Model file for the job. Use its own axes, mm. Face numbers are marked on the shaded views. A direction names the side the tool comes from. Coordinates: 2 decimals unless noted, no trailing zeros. Order: outer loops, then holes, each group sorted by start corner. A loop starts at its lowest first (then second) coordinate and runs counter-clockwise, first axis right, second up. Notation, with made-up numbers: M 23.25,-39.5 L 72.25,-39.5 A31 cw 72.25,-6.5 Z; hole C 12,0 d11. An arc over 180 degrees is marked long. Return JSON: item names as keys, results as strings.
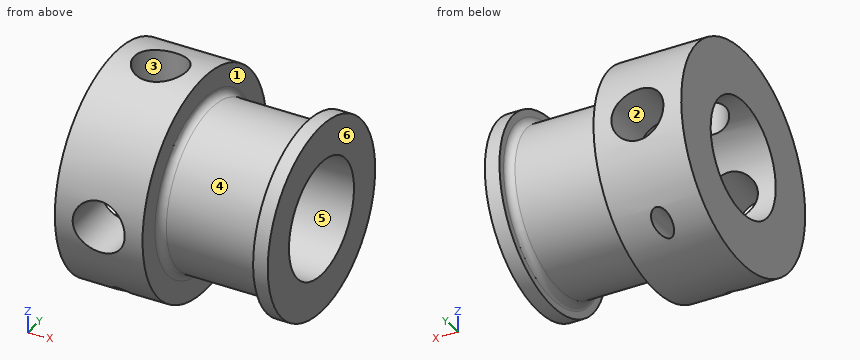
```python
from build123d import *

# Parameters (mm, degrees)
SKETCH1_R            = 4.7625
SKETCH1_R_2          = 2.499995
BASE_DEPTH           = 8.89
CRIMPHOLE_DEPTH      = 12.153246725
CRIMPHOLE_DEPTH_BACK = 12.153246725
SKETCH7_R            = 0.396875
SKETCH3_W            = 1.1303
SKETCH3_H            = 4.7635
CUTTERRAD_R          = 0.3175
CIRPATTERN1_COUNT    = 4


with BuildPart() as part:
    # Sketch1 → Base (new body)
    with BuildSketch(Plane(origin=(0, 0, 0), x_dir=(0, 0, -1), z_dir=(1, 0, 0))):
        Circle(SKETCH1_R)
        Circle(SKETCH1_R_2, mode=Mode.SUBTRACT)
    extrude(amount=BASE_DEPTH)

    # Sketch2 → Spool (revolve, cut)
    with BuildSketch(Plane.XY, mode=Mode.PRIVATE) as spool_sk:
        Polygon((3.81, 4.7625), (8.89, 4.7625), (8.89, 4.1275), (8.255, 4.1275), (8.255, 3.4925), (3.81, 3.4925), align=None)
    revolve(spool_sk.sketch.rotate(Axis((8.89, 0, 0), (-1, 0, 0)), 90), axis=Axis((8.89, 0, 0), (-1, 0, 0)), mode=Mode.SUBTRACT)

    # Sketch7 → CrimpHole (cut, two sides: drawn at the far end of the back side and taken through both)
    with BuildSketch(Plane(origin=(0, 0, 0), x_dir=(1, 0, 0), z_dir=(0, 1, 0)).offset(-CRIMPHOLE_DEPTH_BACK)):
        with Locations(Location((1.905, 3.81, 0), (0, 0, 270))):
            Circle(SKETCH7_R)
    extrude(amount=CRIMPHOLE_DEPTH + CRIMPHOLE_DEPTH_BACK, mode=Mode.SUBTRACT)

    # Sketch3 → ShaftSetScrew (revolve, cut)
    with BuildSketch(Plane.YZ.offset(1.905)):
        with Locations((0.56515, 2.38175)):
            Rectangle(SKETCH3_W, SKETCH3_H)
    shaftsetscrew = revolve(axis=Axis((1.905, 0, -6.35), (0, 0, 1)), mode=Mode.SUBTRACT)

    # CutterRad
    cutterrad_edges = [part.edges().sort_by_distance(p)[0] for p in [
        (3.81, 0, 3.4925),
        (8.255, 0, 3.4925),
    ]]
    fillet(cutterrad_edges, radius=CUTTERRAD_R)

    # CirPattern1: ShaftSetScrew ×4 about axis, 1 skipped
    cirpattern1_axis = Axis((8.89, 0, 0), (-1, 0, 0))
    add([shaftsetscrew.rotate(cirpattern1_axis, i * 360 / CIRPATTERN1_COUNT) for i in range(1, CIRPATTERN1_COUNT) if i not in (2,)], mode=Mode.SUBTRACT)


solid = part.part
```
Item 1: Saw through at A-A (z = 0). Count the separate pieces of the cut face and the enclosed holes in it, and give its area (3 significant figures).
Check result:
{"separate pieces": "4", "enclosed holes": "0", "area": "18.0 mm2"}
Item 2: 3-axis set-ups, long thin cutter, end or side, ignore diameter. For the marked faces 1 and 2: which of +Z, -Z, +X, -X, +Y, -Y reach the whole face in a straight line?
Check result:
{"face 1": "none", "face 2": "+Y, -Y"}
Item 3: Wall check: line 1 (Y direction, x = 3.75, z = 0); line 2 (X direction, y = -2.75, z = 0); line 3 (Y direction, x = 4.25, z = 1). Give the ranges that are in metal, low to high.
Check result:
{"line 1": "y = -4.76 to -2.5, 2.5 to 4.76", "line 2": "x = 0 to 0.77, 3.04 to 8.89", "line 3": "y = -3.35 to -2.29, 2.29 to 3.35"}
Item 4: Pull direction Y, two halves, no side cores. Call the marked faces 3, 4, 5 and 6: +Y half, -Y half, draft (parallel to the pull), parting line (faces both ways), or undercut.
Check result:
{"face 3": "undercut", "face 4": "parting line", "face 5": "undercut", "face 6": "draft"}
Item 5: Saw through at B-B (x = 4.75). Write the cut outline in (y, z) (1 decimal).
Check result:
{"outline": "C 0,0 d7; hole C 0,0 d5"}
Item 6: Drop flat-ended pins along their axis: pin 1 Ø1 at (x, z) = (1.5, -1) entering from +Y; pin 2 Ø1.5 at (x, z) = (6.5, 0) entering from +Y; pin 3 Ø1 at (x, z) = (7.5, 3.5) entering from -Y. Give the stop position or say it passes through.
Check result:
{"pin 1": "stops at y = 4.7", "pin 2": "stops at y = 3.49", "pin 3": "stops at y = -1.79"}
